For this review, use the dimensioned drawing (mm, ordinates from the lowest corner) and the shaded views. A direction names the side the tool comes from. Coordinates: 2 decimals unless noted, no trailing zeros. Loops run counter-clockwise (first coordinate to the right, second up) from the corner with the lowest first, then second, coordinate; pieces in that order, holes last. Notation, with made-up numbers: (-5, 33.25) - (24, 33.25) arc R11 cw to (24, 45.25) - close; hole circle Ø4 at (-35.75, 34). An arc over 180 degrees is marked (long way). One line per item, written item: value. Start each with the question number.
1. Insertion check: P1, Ø6, axis at x = 7.75, z = 7.5, coming from the -Y side; P2, Ø4, axis at x = 92.25, z = 7.5, coming from the -Y side; P3, Ø1, axis at x = 82.5, z = 1.5, coming from the +Y side. Each pin has a flat end and moves straight along its axis. Give the tip position at first contact, or say it passes through.
2. For the marked faces 1 and 2, list the 3-axis set-ups (+Z, -Z, +X, -X, +Y, -Y) from which the entire face can be reached by the end or side of a thin tool; tool diameter is ignored.
3. We need section D-D, the plane z = 14. Give the boundary of the cut face in (x, y).
4. To check wall thickness, follow line 1 (Z direction, x = 92.25, y = 1.7); line 2 (Z direction, x = 77, y = 1); line 3 (X direction, y = 2.6, z = 13.25). State the ranges of each line that lie inside material, in increasing order.
5. We need section B-B, the plane z = 7.5. Give the boundary of the cut face in (x, y).
6. We need section A-A, the plane y = 2.7. Give the boundary of the cut face in (x, z), then the cut area to 3 significant figures.
7. We need section C-C, the plane x = 67.5. Give the boundary of the cut face in (y, z).
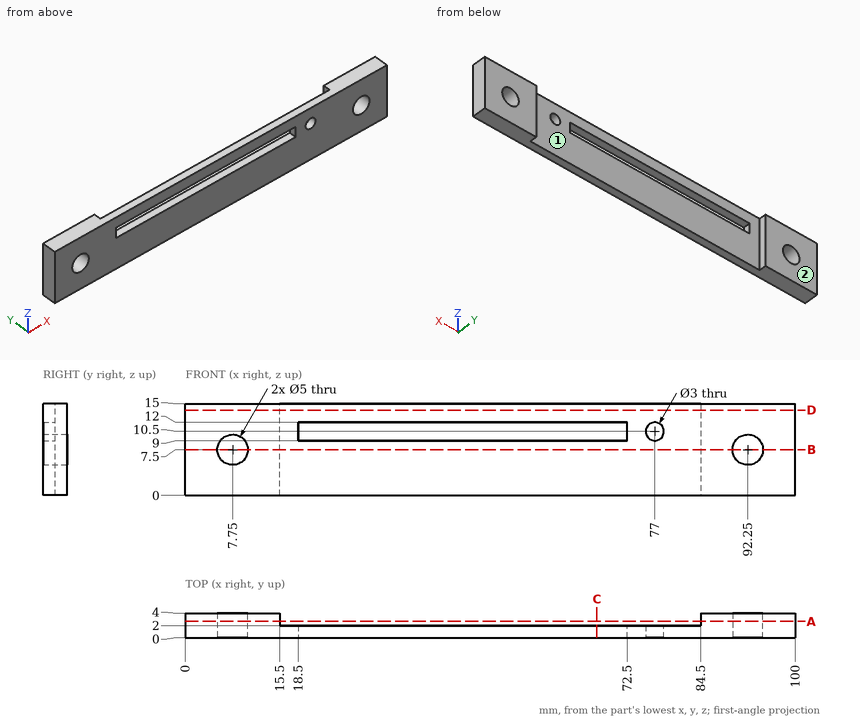
Findings below:
1. P1: y = 0
1. P2: through
1. P3: y = 2
2. face 1: +Z, -Z, +Y
2. face 2: +Z, -Z, +X, -X, +Y
3. outline: (0, 0) - (100, 0) - (100, 4) - (84.5, 4) - (84.5, 2) - (15.5, 2) - (15.5, 4) - (0, 4) - close
4. line 1: 0 to 5, 10 to 15
4. line 2: 0 to 9, 12 to 15
4. line 3: 0 to 15.5, 84.5 to 100
5. outline: (0, 0) - (5.25, 0) - (5.25, 4) - (0, 4) - close; (10.25, 0) - (89.75, 0) - (89.75, 4) - (84.5, 4) - (84.5, 2) - (15.5, 2) - (15.5, 4) - (10.25, 4) - close; (94.75, 0) - (100, 0) - (100, 4) - (94.75, 4) - close
6. outline: (0, 0) - (15.5, 0) - (15.5, 15) - (0, 15) - close; (84.5, 0) - (100, 0) - (100, 15) - (84.5, 15) - close; hole circle Ø5 at (7.75, 7.5); hole circle Ø5 at (92.25, 7.5)
6. area: 426 mm2
7. outline: (0, 0) - (2, 0) - (2, 9) - (0, 9) - close; (0, 12) - (2, 12) - (2, 15) - (0, 15) - close
